Geometry: final body of the model. Coordinates: model frame, mm. Face numbers are marked on the shaded views. A direction names the side the tool comes from. Coordinates: 2 decimals unless noted, no trailing zeros. Order: outer loops, then holes, each group sorted by start corner. A loop starts at its lowest first (then second) coordinate and runs counter-clockwise, first axis right, second up. Notation, with made-up numbers: (58, -2) -> (72, -2) arc R15 ccw to (72, 27) -> close; hole circle Ø1 at (12, 30). An arc over 180 degrees is marked (long way). Use CSV: the item, a comma, the result in double quotes. Start each with the question number.
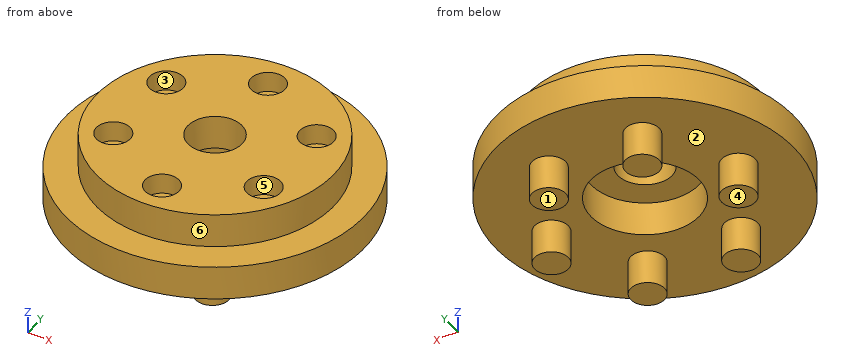
from build123d import *

# Parameters (mm, degrees)
SKETCH2_R             = 2.5
BOSS_EXTRUDE1_DEPTH   = 5
BOSS_EXTRUDE1_2_DEPTH = 5
BOSS_EXTRUDE1_3_DEPTH = 5
BOSS_EXTRUDE1_4_DEPTH = 5
BOSS_EXTRUDE1_5_DEPTH = 5
BOSS_EXTRUDE1_6_DEPTH = 5
SKETCH3_R             = 22
BOSS_EXTRUDE2_DEPTH   = 5
SKETCH4_R             = 17.5
BOSS_EXTRUDE3_DEPTH   = 5
SKETCH5_R             = 8
CUT_EXTRUDE1_DEPTH    = 10
SKETCH11_R            = 2.5
CUT_EXTRUDE4_DEPTH    = 3
SKETCH13_R            = 8
SKETCH13_R_2          = 4
BOSS_EXTRUDE5_DEPTH   = 5


with BuildPart() as part:
    # Sketch2 → Boss-Extrude1 (new body)
    with BuildSketch(Plane.XY):
        with Locations((-7, 12.124355653)):
            Circle(SKETCH2_R)
    extrude(amount=BOSS_EXTRUDE1_DEPTH)



with BuildPart() as body_2:
    # Sketch2 → Boss-Extrude1 2 (new body)
    with BuildSketch(Plane.XY):
        with Locations((7, 12.124355653)):
            Circle(SKETCH2_R)
    extrude(amount=BOSS_EXTRUDE1_2_DEPTH)


with BuildPart() as body_3:
    # Sketch2 → Boss-Extrude1 3 (new body)
    with BuildSketch(Plane.XY):
        with Locations((14, 0)):
            Circle(SKETCH2_R)
    extrude(amount=BOSS_EXTRUDE1_3_DEPTH)


with BuildPart() as body_4:
    # Sketch2 → Boss-Extrude1 4 (new body)
    with BuildSketch(Plane.XY):
        with Locations((7, -12.124355653)):
            Circle(SKETCH2_R)
    extrude(amount=BOSS_EXTRUDE1_4_DEPTH)


with BuildPart() as body_5:
    # Sketch2 → Boss-Extrude1 5 (new body)
    with BuildSketch(Plane.XY):
        with Locations((-7, -12.124355653)):
            Circle(SKETCH2_R)
    extrude(amount=BOSS_EXTRUDE1_5_DEPTH)


with BuildPart() as body_6:
    # Sketch2 → Boss-Extrude1 6 (new body)
    with BuildSketch(Plane.XY):
        with Locations((-14, 0)):
            Circle(SKETCH2_R)
    extrude(amount=BOSS_EXTRUDE1_6_DEPTH)


with BuildPart() as part_1:
    add(part.part)

    add(body_2.part)  # Boss-Extrude2 merges body 2

    add(body_3.part)  # Boss-Extrude2 merges body 3

    add(body_4.part)  # Boss-Extrude2 merges body 4

    add(body_5.part)  # Boss-Extrude2 merges body 5

    add(body_6.part)  # Boss-Extrude2 merges body 6
    # Sketch3 → Boss-Extrude2 (add)
    with BuildSketch(Plane.XY.offset(5)):
        Circle(SKETCH3_R)
    extrude(amount=BOSS_EXTRUDE2_DEPTH)

    # Sketch4 → Boss-Extrude3 (add)
    with BuildSketch(Plane.XY.offset(10)):
        Circle(SKETCH4_R)
    extrude(amount=BOSS_EXTRUDE3_DEPTH)

    # Sketch5 → Cut-Extrude1 (cut)
    with BuildSketch(Plane.XY.offset(15)):
        Circle(SKETCH5_R)
    extrude(amount=-CUT_EXTRUDE1_DEPTH, mode=Mode.SUBTRACT)

    # Sketch11 → Cut-Extrude4 (cut)
    with BuildSketch(Plane.XY.offset(15)):
        with Locations((0, 13)):
            Circle(SKETCH11_R)
        with Locations((11.258330249, 6.5)):
            Circle(SKETCH11_R)
        with Locations((11.258330249, -6.5)):
            Circle(SKETCH11_R)
        with Locations((0, -13)):
            Circle(SKETCH11_R)
        with Locations((-11.258330249, -6.5)):
            Circle(SKETCH11_R)
        with Locations((-11.258330249, 6.5)):
            Circle(SKETCH11_R)
    extrude(amount=-CUT_EXTRUDE4_DEPTH, mode=Mode.SUBTRACT)

    # Sketch13 → Boss-Extrude5 (add)
    with BuildSketch(Plane.XY.offset(15)):
        Circle(SKETCH13_R)
        Circle(SKETCH13_R_2, mode=Mode.SUBTRACT)
    extrude(amount=-BOSS_EXTRUDE5_DEPTH)


solid = part_1.part
(1) Access query for the marked faces 1, 2 and 3. Directions: +Z, -Z, +X, -X, +Y, -Y. A direction counts if a zero-diameter tool reaches every point of the face in a straight line with its end or side. Return the directions, or none.
(2) Section D-D (z = 2.25). Return loops of the section in (x, y).
(3) Section A-A (y = 0). Return loops of the section in (x, z).
(4) Line query: line 1 (Y direction, x = -11.5, z = 13); line 2 (Z direction, x = -8.5, y = 20); line 3 (Y direction, x = 5.5, z = 7). Output: solid intervals per line, ascending. Write a range as from..to.
(5) First-contact query: pin 1 (6.5 mm diameter, centred on x = 0, y = 0, fed in from -Z); pin 2 (3 mm diameter, centred on x = -17, z = 5.5, fed in from -Y); pin 3 (2 mm diameter, centred on x = -10, y = 6, fed in from -Z); pin 4 (8 mm diameter, centred on x = -5, z = 11.5, fed in from -Y). Flat tips, straight axial feed; report the tip coordinate or a pass-through.
(6) Section C-C (y = 6.5). Return loops of the section in (x, z).
(7) Mould query, pull axis Y, two halves, no side actions, for the marked faces 4, 5 and 6. Classes: pulls with the +Y half, pulls with the -Y half, needs draft (parallel to the pull), parting line crosses it, or undercut.
(8) Section B-B (x = 7). Return loops of the section in (y, z).
Check sheet entries:
1,face 1,"-Z, +X, -X, +Y, -Y"
1,face 2,"-Z"
1,face 3,"+Z"
2,outline,"circle Ø5 at (-14, 0); circle Ø5 at (-7, -12.12); circle Ø5 at (-7, 12.12); circle Ø5 at (7, -12.12); circle Ø5 at (7, 12.12); circle Ø5 at (14, 0)"
3,outline,"(-22, 5) -> (-16.5, 5) -> (-16.5, 0) -> (-11.5, 0) -> (-11.5, 5) -> (-8, 5) -> (-8, 10) -> (-4, 10) -> (-4, 15) -> (-17.5, 15) -> (-17.5, 10) -> (-22, 10) -> close; (4, 10) -> (8, 10) -> (8, 5) -> (11.5, 5) -> (11.5, 0) -> (16.5, 0) -> (16.5, 5) -> (22, 5) -> (22, 10) -> (17.5, 10) -> (17.5, 15) -> (4, 15) -> close"
4,line 1,"y = -13.19..-8.99, -4.01..4.01, 8.99..13.19"
4,line 2,"z = 5..10"
4,line 3,"y = -21.3..-5.81, 5.81..21.3"
5,pin 1,"passes through"
5,pin 2,"stops at y = -15.61"
5,pin 3,"stops at z = 5"
5,pin 4,"stops at y = -21.96"
6,outline,"(-21.02, 5) -> (-4.66, 5) -> (-4.66, 10) -> (4.66, 10) -> (4.66, 5) -> (21.02, 5) -> (21.02, 10) -> (16.25, 10) -> (16.25, 15) -> (13.76, 15) -> (13.76, 12) -> (8.76, 12) -> (8.76, 15) -> (-8.76, 15) -> (-8.76, 12) -> (-13.76, 12) -> (-13.76, 15) -> (-16.25, 15) -> (-16.25, 10) -> (-21.02, 10) -> close"
7,face 4,"needs draft"
7,face 5,"undercut"
7,face 6,"parting line crosses it"
8,outline,"(-20.86, 5) -> (-14.62, 5) -> (-14.62, 0) -> (-9.62, 0) -> (-9.62, 5) -> (-3.87, 5) -> (-3.87, 10) -> (3.87, 10) -> (3.87, 5) -> (9.62, 5) -> (9.62, 0) -> (14.62, 0) -> (14.62, 5) -> (20.86, 5) -> (20.86, 10) -> (16.04, 10) -> (16.04, 15) -> (-16.04, 15) -> (-16.04, 10) -> (-20.86, 10) -> close"
